```python
from build123d import *

# Parameters (mm, degrees)
SKETCH1_R           = 2.6035
BOSS_EXTRUDE1_DEPTH = 12.7


with BuildPart() as part:
    # Sketch1 → Boss-Extrude1 (new body)
    with BuildSketch(Plane(origin=(0, 0, 0), x_dir=(1, 0, 0), z_dir=(0, 1, 0))):
        with BuildLine():
            Line((6.35, -3.666174209), (6.35, -58.718791294))
            ThreePointArc((6.35, -58.718791294), (0, -59.31849574), (-6.35, -58.718791294))
            Line((-6.35, -58.718791294), (-6.35, -3.666174209))
            Line((-6.35, -3.666174209), (-54.02696494, 23.860134333))
            ThreePointArc((-54.02696494, 23.860134333), (-51.371324225, 29.65924787), (-47.67696494, 34.858656961))
            Line((-47.67696494, 34.858656961), (0, 7.332348419))
            Line((0, 7.332348419), (47.67696494, 34.858656961))
            ThreePointArc((47.67696494, 34.858656961), (51.371324225, 29.65924787), (54.02696494, 23.860134333))
            Line((54.02696494, 23.860134333), (6.35, -3.666174209))
        make_face()
        with Locations(Location((0, -25.4, 0), (0, 0, 270))):
            Circle(SKETCH1_R, mode=Mode.SUBTRACT)
        with Locations(Location((-21.997045256, 12.7, 0), (0, 0, 270))):
            Circle(SKETCH1_R, mode=Mode.SUBTRACT)
        with Locations(Location((21.997045256, 12.7, 0), (0, 0, 270))):
            Circle(SKETCH1_R, mode=Mode.SUBTRACT)
    extrude(amount=BOSS_EXTRUDE1_DEPTH)


solid = part.part
```
For this review, take the finished solid that the model builds, in its own axes (mm). A direction names the side the tool comes from. Coordinates: 2 decimals unless noted, no trailing zeros. Order: outer loops, then holes, each group sorted by start corner. A loop starts at its lowest first (then second) coordinate and runs counter-clockwise, first axis right, second up. Notation, with made-up numbers: (87, 89.5) - (122, 89.5) arc R37 cw to (122, 127.5) - close; hole circle Ø2 at (75.5, -3.5). An arc over 180 degrees is marked (long way). Answer as a JSON object with one key per item and string values. Group by question number.
1. The part is to be moulded in two halves that separate along X. For faces 1 (the cylindrical face through (0.782, 6.261, 27.883)), 2 (the cylindrical face through (51.327, 6.261, -29.737)), 3 (the flat face through (0, 0, 2)), say which applies: pulls with the +X half, pulls with the -X half, needs draft (parallel to the pull), parting line crosses it, or undercut.
2. We need section D-D on z = 51. State the section outline as (x, y) points.
3. We need section C-C on z = -12.7. State the section outline as (x, y) points.
4. We need section A-A on z = 25.4. State the section outline as (x, y) points, then the cut area to 3 significant figures.
5. Clearance check with flat-ended pins moving along their axes: P1, Ø6, axis at y = 7.5, z = 8.5, coming from the +X side; P2, Ø6, axis at x = -41.5, y = 6, coming from the +Z side; P3, Ø4, axis at x = 16.5, y = 8, coming from the +Z side. State where each tip first meets the part, or that it passes through.
6. We need section B-B on y = 1.5. State the section outline as (x, z) points.
7. For faces 4 (the cylindrical face through (-51.416, 6.261, -29.582)), 5 (the flat face through (-6.35, 6, 32)), 6 (the flat face through (-24.172, 6.261, -21.288)), 7 (the flat face through (6.35, 6, 31)), list the 3-axis set-ups (+Z, -Z, +X, -X, +Y, -Y) from which the entire face can be reached by the end or side of a thin tool; tool diameter is ignored.
8. For probe 1 along X at (y, z) = (9.5, 25.4); probe 2 along X at (y, z) = (12.25, -11); probe 3 along X at (y, z) = (3.5, -12.7), list the stretches that pass through material, from the lowest coordinate up.
Final values:
{
 "1": {"face 1": "undercut", "face 2": "pulls with the +X half", "face 3": "needs draft"},
 "2": {"outline": "(-6.35, 0) - (6.35, 0) - (6.35, 12.7) - (-6.35, 12.7) - close"},
 "3": {"outline": "(-34.7, 0) - (-24.6, 0) - (-24.6, 12.7) - (-34.7, 12.7) - close; (-19.39, 0) - (-9.3, 0) - (-9.3, 12.7) - (-19.39, 12.7) - close; (9.3, 0) - (19.39, 0) - (19.39, 12.7) - (9.3, 12.7) - close; (24.6, 0) - (34.7, 0) - (34.7, 12.7) - (24.6, 12.7) - close"},
 "4": {"outline": "(-6.35, 0) - (-2.6, 0) - (-2.6, 12.7) - (-6.35, 12.7) - close; (2.6, 0) - (6.35, 0) - (6.35, 12.7) - (2.6, 12.7) - close", "area": "95.2 mm²"},
 "5": {"P1": "x = 6.35", "P2": "z = -14.9", "P3": "z = -1.04"},
 "6": {"outline": "(-54.03, -23.86) arc R33.92 ccw to (-47.68, -34.86) - (0, -7.33) - (47.68, -34.86) arc R33.92 ccw to (54.03, -23.86) - (6.35, 3.67) - (6.35, 58.72) arc R33.92 ccw to (-6.35, 58.72) - (-6.35, 3.67) - close; hole circle Ø5.21 at (-22, -12.7); hole circle Ø5.21 at (0, 25.4); hole circle Ø5.21 at (22, -12.7)"},
 "7": {"face 4": "-Z, -X, +Y, -Y", "face 5": "+Z, -X, +Y, -Y", "face 6": "-Z, +Y, -Y", "face 7": "+Z, +X, +Y, -Y"},
 "8": {"probe 1": "-6.35 to -2.6, 2.6 to 6.35", "probe 2": "-31.75 to -23.97, -20.03 to -6.35, 6.35 to 20.03, 23.97 to 31.75", "probe 3": "-34.7 to -24.6, -19.39 to -9.3, 9.3 to 19.39, 24.6 to 34.7"}
}
